Can you work these out from the drawing? Everything is in mm from the part's minimum corner. A direction names the side the tool comes from. Round coordinates to 2 decimals unless told otherwise and drop trailing zeros. Write each loop counter-clockwise with the first axis right and the second up, starting at its lowest first coordinate (ties: lowest second). Pieces come first, ordered by that corner, then holes. Notation, with made-up numbers: (-19, -25.5) - (18, -25.5) arc R27 cw to (18, -3.5) - close; hole circle Ø10 at (62, 30.5). An arc over 180 degrees is marked (long way). One line per item, written item: value. Start each with the question number.
(1) I want a section at D-D on z = 56.5. List the corners of the cut face in (x, y) for me, plus the area to 3 significant figures.
(2) I'm going to push flat-ended pins straight in: pin 1 Ø10 at (y, z) = (7.5, 27.5) entering from +X; pin 2 Ø3 at (x, y) = (15.5, 9) entering from -Z. Where does each tip first touch, or does it pass through?
(3) I want a section at C-C on x = 17.5. List the corners of the cut face in (y, z) for me, plus the area to 3 significant figures.
(4) On a 3-axis mill with a long thin cutter (end or side, diameter ignored), from which of +Z, -Z, +X, -X, +Y, -Y can I reach the whole of each face in a straight line? I mean the marked faces 1 and 2. Say none if no direction works.
(5) I want a section at B-B on z = 34.5. List the corners of the cut face in (x, y) for me, plus the area to 3 significant figures.
(6) If I drill on L1, parallel to X at y = 18.75, z = 35; L2, parallel to Z at x = 18.25, y = 9; L3, parallel to Z at x = 13.25, y = 10, over which ranges is the centre line in solid material (lowest first)? Write a range as from..to.
(7) I want a section at A-A on y = 9.5. List the corners of the cut face in (x, z) for me, plus the area to 3 significant figures.
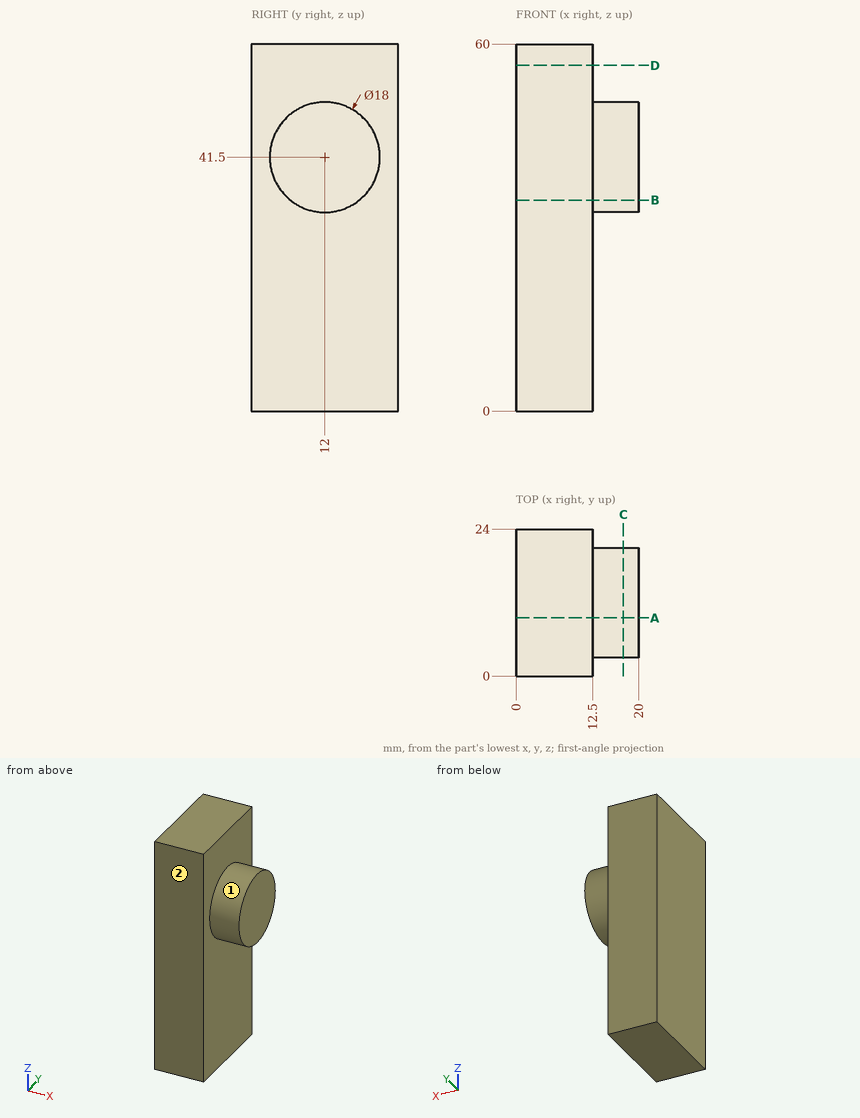
Established:
1. outline: (0, 0) - (12.5, 0) - (12.5, 24) - (0, 24) - close
1. area: 300 mm2
2. pin 1: x = 12.5
2. pin 2: z = 32.63
3. outline: circle Ø18 at (12, 41.5)
3. area: 254 mm2
4. face 1: +X
4. face 2: +Z, -Z, +X, -X, -Y
5. outline: (0, 0) - (12.5, 0) - (12.5, 6.34) - (20, 6.34) - (20, 17.66) - (12.5, 17.66) - (12.5, 24) - (0, 24) - close
5. area: 385 mm2
6. L1: 0..12.5
6. L2: 33.01..49.99
6. L3: 32.73..50.27
7. outline: (0, 0) - (12.5, 0) - (12.5, 32.85) - (20, 32.85) - (20, 50.15) - (12.5, 50.15) - (12.5, 60) - (0, 60) - close
7. area: 880 mm2
